Verification items for the finished model (mm, model axes). Face numbers are marked on the shaded views. A direction names the side the tool comes from. Round coordinates to 2 decimals unless told otherwise and drop trailing zeros. Order: outer loops, then holes, each group sorted by start corner. A loop starts at its lowest first (then second) coordinate and runs counter-clockwise, first axis right, second up. Notation, with made-up numbers: (7.5, 42.5) -> (35.5, 42.5) arc R18 ccw to (35.5, 57.5) -> close; hole circle Ø10 at (-10, 41.25). An arc over 180 degrees is marked (long way). Return JSON: item names as keys, results as strings. Group by question number.
1) Draft check along Y on the marked faces 5, 6 and 7. Enter one of: pulls with the +Y half, pulls with the -Y half, needs draft (parallel to the pull), parting line crosses it, or undercut.
2) Section check B-B on x = -11. Enter the section's corners in (y, z).
3) Section check A-A on x = -40. Enter the section's corners in (y, z).
4) Scan lines: L1, parallel to Y at x = -30, z = 77; L2, parallel to Y at x = -7, z = 114; L3, parallel to Z at x = -11.5, y = 0. Record each from-to range of solid material in increasing order.
5) Section check C-C on x = -53. Enter the section's corners in (y, z).
6) Tool access check on the marked faces 1, 2, 3 and 4. Record the directions out of +Z, -Z, +X, -X, +Y, -Y that give a thin tool (end or side, any length) a straight path to the whole face; none if there is none.
7) Section check D-D on z = 34.5. Enter the section's corners in (x, y), plus the area to 3 significant figures.
8) Depth check by flat-ended pin: pin 1 (3 mm diameter, centred on y = -48, z = 129, fed in from +X); pin 2 (5 mm diameter, centred on y = 40, z = 100.5, fed in from -X); pin 3 (20.5 mm diameter, centred on x = -41.5, z = 80, fed in from -Y); pin 4 (12.5 mm diameter, centred on x = -32, z = 71.5, fed in from +Y). Enter the tip coordinate at first touch or a pass-through.
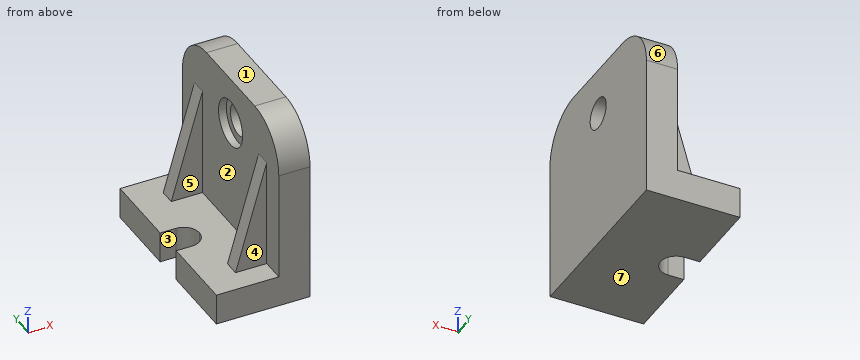
```python
from build123d import *

# Parameters (mm, degrees)
F1_DEPTH  = 76.2
F2_R      = 12.7
F3_DEPTH  = 76.201
F5_DEPTH  = 46.736
F6_R      = 19.05
F7_DEPTH  = 6.35
F8_R      = 38.1
F11_DEPTH = 12.7


# Not quite as in the source:
# - a pattern or mirror of a feature is missing from the dataset's text; its kind, count and spacing are read off the source's solid


with BuildPart() as f1:
    # F0 (on Front) → F1 (new body, symmetric)
    with BuildSketch(Plane.XZ):
        Polygon((-76.2, 0), (0, 0), (0, 152.4), (-25.4, 152.4), (-25.4, 25.4), (-76.2, 25.4), align=None)
    extrude(amount=F1_DEPTH, both=True)

    # F2 (on Right) → F3 (cut, through all)
    with BuildSketch(Plane.YZ):
        with Locations((0, 114.3)):
            Circle(F2_R)
    extrude(amount=-F3_DEPTH, mode=Mode.SUBTRACT)

    # F4 (on face) → F5 (cut)
    with BuildSketch(Plane.XY.offset(25.4)):
        with BuildLine():
            ThreePointArc((-63.5, -12.7), (-54.5197438789, -8.9802561211), (-50.8, 0))
            ThreePointArc((-50.8, 0), (-54.5197438789, 8.9802561211), (-63.5, 12.7))
            Line((-63.5, 12.7), (-76.2, 12.7))
            Line((-76.2, 12.7), (-76.2, -12.7))
            Line((-76.2, -12.7), (-63.5, -12.7))
        make_face()
    extrude(amount=-F5_DEPTH, mode=Mode.SUBTRACT)

    # F6 (on face) → F7 (cut)
    with BuildSketch(Plane(origin=(-25.4, 0, 0), x_dir=(0, -1, 0), z_dir=(-1, 0, 0))):
        with Locations((-0.0589386239, 113.8949071477)):
            Circle(F6_R)
    extrude(amount=-F7_DEPTH, mode=Mode.SUBTRACT)

    # F8
    f8_edges = [f1.edges().sort_by_distance(p)[0] for p in [
        (-12.7, 76.2, 152.4),
        (-12.7, -76.2, 152.4),
    ]]
    fillet(f8_edges, radius=F8_R)

    # F10 (on offset) → F11 (join)
    with BuildSketch(Plane.XZ.offset(44.45)):
        Polygon((-25.4, 25.4), (-25.4, 114.3), (-50.8, 25.4), align=None)
    f11 = extrude(amount=F11_DEPTH)

    # F11_copies: F11 across plane
    add(f11.mirror(Plane.ZX))


solid = f1.part
```
Check result:
{
 "1": {"face 5": "undercut", "face 6": "pulls with the +Y half", "face 7": "needs draft"},
 "2": {"outline": "(-76.2, 0) -> (76.2, 0) -> (76.2, 114.3) arc R38.1 ccw to (38.1, 152.4) -> (-38.1, 152.4) arc R38.1 ccw to (-76.2, 114.3) -> close; hole circle Ø25.4 at (0, 114.3)"},
 "3": {"outline": "(-76.2, 0) -> (76.2, 0) -> (76.2, 25.4) -> (57.15, 25.4) -> (57.15, 63.2) -> (44.45, 63.2) -> (44.45, 25.4) -> (-44.45, 25.4) -> (-44.45, 63.2) -> (-57.15, 63.2) -> (-57.15, 25.4) -> (-76.2, 25.4) -> close"},
 "4": {"L1": "-57.15 to -44.45, 44.45 to 57.15", "L2": "-76.2 to -12.7, 12.7 to 76.2", "L3": "0 to 101.6, 127 to 152.4"},
 "5": {"outline": "(-76.2, 0) -> (-7.14, 0) -> (-7.14, 25.4) -> (-76.2, 25.4) -> close; (7.14, 0) -> (76.2, 0) -> (76.2, 25.4) -> (7.14, 25.4) -> close"},
 "6": {"face 1": "+Z, +X, -X, +Y, -Y", "face 2": "+Z, -X", "face 3": "+Z, -Z, -X", "face 4": "+Z, -X, -Y"},
 "7": {"outline": "(-48.2, -57.15) -> (-25.4, -57.15) -> (-25.4, -76.2) -> (0, -76.2) -> (0, 76.2) -> (-25.4, 76.2) -> (-25.4, 57.15) -> (-48.2, 57.15) -> (-48.2, 44.45) -> (-25.4, 44.45) -> (-25.4, -44.45) -> (-48.2, -44.45) -> close", "area": "4,450 mm^2"},
 "8": {"pin 1": "x = 0", "pin 2": "x = -25.4", "pin 3": "y = -57.15", "pin 4": "y = 57.15"}
}
